from build123d import *

# Parameters (mm, degrees)
SKETCH_2_R          = 2.5
EXTRUDE_1_DEPTH     = 8
SKETCH_9_R          = 2.25
CUT_EXTRUDE_6_DEPTH = 2
SKETCH_10_R         = 1.725
EXTRUDE_3_DEPTH     = 4
FILLET_9_R          = 1
FILLET_6_R          = 1
FILLET_11_R         = 0.5


with BuildPart() as part:
    # 스케치2 → 보스-돌출1 (new body)
    with BuildSketch(Plane.XY):
        with BuildLine():
            Line((8.317867543, 16.224371176), (13.7243035, 16.224371176))
            Line((13.7243035, 16.224371176), (15.084656802, 16.224371176))
            Line((15.084656802, 16.224371176), (15.084656802, 8.724371176))
            ThreePointArc((15.084656802, 8.724371176), (15.309326229, 8.092815555), (15.882381806, 7.745042413))
            Line((15.882381806, 7.745042413), (17.349168707, 7.442085607))
            ThreePointArc((17.349168707, 7.442085607), (17.461588205, 7.375174839), (17.508595785, 7.253086831))
            ThreePointArc((17.508595785, 7.253086831), (17.192711955, 4.187660486), (16.059003603, 1.322119239))
            ThreePointArc((16.059003603, 1.322119239), (15.315387006, 0.571939712), (14.29334298, 0.305179564))
            Line((14.29334298, 0.305179564), (12.864118803, 0.322230851))
            ThreePointArc((12.864118803, 0.322230851), (9.906475316, -2.49254573), (8.205466836, -6.204309777))
            ThreePointArc((8.205466836, -6.204309777), (6.437083645, -10.39249276), (1.899177239, -10.667194879))
            Line((1.899177239, -10.667194879), (-2.713922879, -9.439136425))
            Line((-2.713922879, -9.439136425), (-6.086658366, -8.506851574))
            ThreePointArc((-6.086658366, -8.506851574), (-8.323670203, -7.337653763), (-9.881865945, -5.351886527))
            Line((-9.881865945, -5.351886527), (-11.641875294, -1.739829609))
            ThreePointArc((-11.641875294, -1.739829609), (-11.678836202, -0.582101362), (-10.839032567, 0.21566468))
            Line((-10.839032567, 0.21566468), (-7.999803479, 1.214399245))
            ThreePointArc((-7.999803479, 1.214399245), (-7.836289234, 1.256793405), (-7.667972201, 1.271060492))
            Line((-7.667972201, 1.271060492), (-5.969536129, 1.271060492))
            Line((-5.969536129, 1.271060492), (-5.969536129, -2.128939508))
            Line((-5.969536129, -2.128939508), (-3.73592311, -2.128939508))
            Line((-3.73592311, -2.128939508), (5.234762536, 15.024331657))
            Line((5.234762536, 15.024331657), (7.166939789, 15.900622709))
            ThreePointArc((7.166939789, 15.900622709), (7.720069967, 16.141893375), (8.317867543, 16.224371176))
        make_face()
        with Locations((3.179026074, -5.859548474)):
            Circle(SKETCH_2_R, mode=Mode.SUBTRACT)
    extrude(amount=EXTRUDE_1_DEPTH)

    # 스케치9 → 컷-돌출6 (cut)
    with BuildSketch(Plane(origin=(0, 16.224371176, 0), x_dir=(1, 0, 0), z_dir=(0, 1, 0))):
        with Locations(Location((11.317867543, -4, 0), (0, 0, 270))):
            Circle(SKETCH_9_R)
    extrude(amount=-CUT_EXTRUDE_6_DEPTH, mode=Mode.SUBTRACT)

    # 스케치10 → 보스-돌출3 (add)
    with BuildSketch(Plane(origin=(0, 14.224371176, 0), x_dir=(1, 0, 0), z_dir=(0, 1, 0))):
        with Locations(Location((11.317867543, -4, 0), (0, 0, 270))):
            Circle(SKETCH_10_R)
    extrude(amount=EXTRUDE_3_DEPTH)

    # 필렛9
    fillet_9_edges = [part.edges().sort_by_distance(p)[0] for p in [
        (11.317867543, 18.224371176, 2.275),
    ]]
    fillet(fillet_9_edges, radius=FILLET_9_R)

    # 필렛6
    fillet_6_edges = [part.edges().sort_by_distance(p)[0] for p in [
        (0.679026074, -5.859548474, 0),
        (0.679026074, -5.859548474, 8),
    ]]
    fillet(fillet_6_edges, radius=FILLET_6_R)

    # 필렛11
    fillet_11_edges = [part.edges().sort_by_distance(p)[0] for p in [
        (15.084656802, 16.224371176, 4),
    ]]
    fillet(fillet_11_edges, radius=FILLET_11_R)


solid = part.part
Design review of the part built by this model. Coordinates are the model's own, in mm. A direction names the side the tool comes from. Round coordinates to 2 decimals unless told otherwise and drop trailing zeros. Write each loop counter-clockwise with the first axis right and the second up, starting at its lowest first coordinate (ties: lowest second). Pieces come first, ordered by that corner, then holes.
Item 1: Wall thickness on L1, parallel to X at y = 15.45, z = 4; L2, parallel to X at y = 15.4, z = 4; L3, parallel to Y at x = 13.75, z = 6.5: over which ranges is each line inside the solid? List them lowest first.
Item 2: Draft analysis for pull direction X (two halves, no side actions). For faces 1 (the flat face through (6.187, 15.456, 3.944)), 2 (the flat face through (3, 3, 0)), 3 (the cylindrical face through (1.195, -7.381, 3.958)), 4 (the cylindrical face through (9.322, 15.238, 5.038)), state which applies: released by +X, released by -X, zero draft, split by the parting line, or undercut.
Item 3: Consider section A-A on y = -0.5. Give the boundary of the cut face in (x, z), and give its area (3 significant figures).
Item 4: For faces 5 (the flat face through (-10.75, -3.57, 3.94)), 6 (the flat face through (15.085, 12, 4)), 7 (the flat face through (0.69, 6.33, 3.94)), list the 3-axis set-ups (+Z, -Z, +X, -X, +Y, -Y) from which the entire face can be reached by the end or side of a thin tool; tool diameter is ignored.
Item 5: Consider section B-B on x = -6.75. Give the boundary of the cut face in (y, z).
Item 6: Consider section C-C on y = 13.25. Give the boundary of the cut face in (x, z).
Item 7: For pin 1 Ø1.5 at (y, z) = (-4.5, 3) entering from -X; pin 2 Ø1.1 at (x, z) = (-4.5, 4.5) entering from +Y; pin 3 Ø2.5 at (y, z) = (0, 6) entering from +X, all flat-tipped, find the tip position at first contact; note any pin that passes through.
Check values:
1. L1: x = 6.17 to 9.07, 9.59 to 13.04, 13.57 to 15.08
1. L2: x = 6.06 to 9.07, 9.59 to 13.04, 13.57 to 15.08
1. L3: y = 0.31 to 16.22
2. face 1: released by -X
2. face 2: zero draft
2. face 3: undercut
2. face 4: undercut
3. outline: (-11.64, 0) - (-5.97, 0) - (-5.97, 8) - (-11.64, 8) - close; (-2.88, 0) - (11.75, 0) - (11.75, 8) - (-2.88, 8) - close
3. area: 162 mm2
4. face 5: +Z, -Z, -X, -Y
4. face 6: +Z, -Z, +X, +Y
4. face 7: +Z, -Z, +Y
5. outline: (-8.28, 0) - (1.27, 0) - (1.27, 8) - (-8.28, 8) - close
6. outline: (4.31, 0) - (15.08, 0) - (15.08, 8) - (4.31, 8) - close
7. pin 1: stops at x = -10.66
7. pin 2: stops at y = -2.13
7. pin 3: stops at x = 16.02
